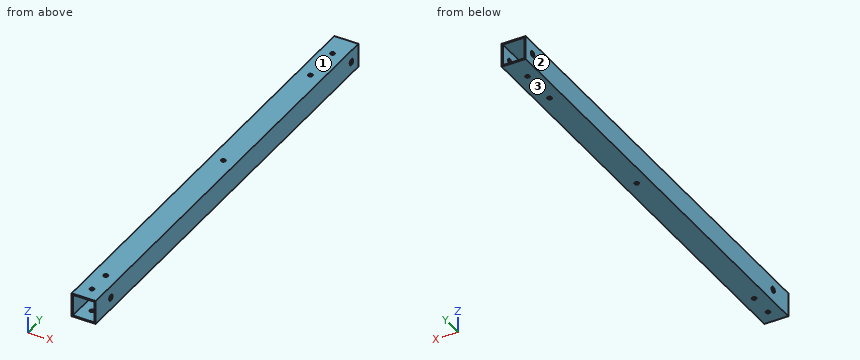
from build123d import *

# Parameters (mm, degrees)
SKETCH1_W           = 25.4
SKETCH1_H           = 25.4
BOSS_EXTRUDE1_DEPTH = 482.6
SKETCH2_R           = 2.286
CUT_EXTRUDE1_DEPTH  = 484.934995635
SKETCH3_R           = 2.286
CUT_EXTRUDE2_DEPTH  = 484.934995635
SKETCH4_R           = 2.286
CUT_EXTRUDE3_DEPTH  = 484.934995635
SKETCH6_R           = 2.286
CUT_EXTRUDE5_DEPTH  = 484.934995635
SKETCH7_R           = 2.286
CUT_EXTRUDE6_DEPTH  = 484.934995635
SKETCH8_R           = 3.175
CUT_EXTRUDE7_DEPTH  = 484.934995635
SKETCH9_R           = 3.175
CUT_EXTRUDE8_DEPTH  = 484.934995635


with BuildPart() as part:
    # Sketch1 → Boss-Extrude1 (new body)
    with BuildSketch(Plane(origin=(0, 0, 0), x_dir=(1, 0, 0), z_dir=(0, 1, 0))):
        with Locations((12.7, 12.7)):
            Rectangle(SKETCH1_W, SKETCH1_H)
        Polygon((1.27, 12.361459156), (1.27, 24.13), (12.7, 24.13), (24.13, 24.13), (24.13, 12.7), (24.13, 1.27), (12.7, 1.27), (1.27, 1.27), align=None, mode=Mode.SUBTRACT)
    extrude(amount=BOSS_EXTRUDE1_DEPTH)

    # Sketch2 → Cut-Extrude1 (cut, through all)
    with BuildSketch(Plane(origin=(0, 0, -25.4), x_dir=(-1, 0, 0), z_dir=(0, 0, -1))):
        with Locations((-12.7, 416.56)):
            Circle(SKETCH2_R)
    extrude(amount=-CUT_EXTRUDE1_DEPTH, mode=Mode.SUBTRACT)

    # Sketch3 → Cut-Extrude2 (cut, through all)
    with BuildSketch(Plane(origin=(0, 0, -25.4), x_dir=(-1, 0, 0), z_dir=(0, 0, -1))):
        with Locations((-12.7, 40.64)):
            Circle(SKETCH3_R)
    extrude(amount=-CUT_EXTRUDE2_DEPTH, mode=Mode.SUBTRACT)

    # Sketch4 → Cut-Extrude3 (cut, through all)
    with BuildSketch(Plane(origin=(0, 0, -25.4), x_dir=(-1, 0, 0), z_dir=(0, 0, -1))):
        with Locations((-12.7, 256.54)):
            Circle(SKETCH4_R)
    extrude(amount=-CUT_EXTRUDE3_DEPTH, mode=Mode.SUBTRACT)

    # Sketch6 → Cut-Extrude5 (cut, through all)
    with BuildSketch(Plane(origin=(0, 0, -25.4), x_dir=(-1, 0, 0), z_dir=(0, 0, -1))):
        with Locations((-12.7, 457.2)):
            Circle(SKETCH6_R)
    extrude(amount=-CUT_EXTRUDE5_DEPTH, mode=Mode.SUBTRACT)

    # Sketch7 → Cut-Extrude6 (cut, through all)
    with BuildSketch(Plane(origin=(0, 0, -25.4), x_dir=(-1, 0, 0), z_dir=(0, 0, -1))):
        with Locations((-12.7, 15.24)):
            Circle(SKETCH7_R)
    extrude(amount=-CUT_EXTRUDE6_DEPTH, mode=Mode.SUBTRACT)

    # Sketch8 → Cut-Extrude7 (cut, through all)
    with BuildSketch(Plane.ZY):
        with Locations((-12.7, 469.9)):
            Circle(SKETCH8_R)
    extrude(amount=-CUT_EXTRUDE7_DEPTH, mode=Mode.SUBTRACT)

    # Sketch9 → Cut-Extrude8 (cut, through all)
    with BuildSketch(Plane.ZY):
        with Locations((-12.7, 27.94)):
            Circle(SKETCH9_R)
    extrude(amount=-CUT_EXTRUDE8_DEPTH, mode=Mode.SUBTRACT)


solid = part.part
Geometry check sheet. Reference: the model listing, model coordinates, mm. Face numbers are marked on the shaded views. Give positions to 0.01 mm unless a question says otherwise; leave off trailing zeros. Write each loop counter-clockwise with the first axis right and the second up, starting at its lowest first coordinate (ties: lowest second). Pieces come first, ordered by that corner, then holes. Notation, with made-up numbers: (38, 35) - (77, 35) arc R22 ccw to (77, 68) - close; hole circle Ø6 at (23, 39). An arc over 180 degrees is marked (long way). Put each result on its own line as item: value.
1. Sectioned sample at B-B, the plane y = 328. Enter the section's corners in (x, z).
Ans:
outline: (0, -25.4) - (25.4, -25.4) - (25.4, 0) - (0, 0) - close; hole (1.27, -24.13) - (24.13, -24.13) - (24.13, -1.27) - (1.27, -1.27) - close
2. Sectioned sample at A-A, the plane x = 19.5. Enter the section's corners in (y, z), plus the area to 3 significant figures.
Ans:
outline: (0, -25.4) - (482.6, -25.4) - (482.6, -24.13) - (0, -24.13) - close; (0, -1.27) - (482.6, -1.27) - (482.6, 0) - (0, 0) - close
area: 1,230 mm²
3. Draft check along Z on the marked faces 1, 2 and 3. Enter one of: +Z half, -Z half, draft (parallel to the pull), parting line (faces both ways), or undercut.
Ans:
face 1: +Z half
face 2: draft
face 3: -Z half
4. Go/stop test with a flat-tipped pin: pin 1 (12 mm diameter, centred on x = 13, z = -19, fed in from -Y). Record where the tip stops, or that it passes through.
Ans:
pin 1: stops at y = 0
5. Thickness scan on line 1 (Y direction, x = 12.7, z = -0.9); line 2 (Y direction, x = 24.45, z = -12.7) (3 decimals); line 3 (Z direction, x = 2.5, y = 434.5). Record the ranges inside material, lowest first.
Ans:
line 1: y = 0 to 12.95, 17.53 to 38.35, 42.93 to 254.25, 258.83 to 414.27, 418.85 to 454.91, 459.49 to 482.6
line 2: y = 0 to 24.765, 31.115 to 466.725, 473.075 to 482.6
line 3: z = -25.4 to -24.13, -1.27 to 0
